Geometry: see drawing. Coordinates: mm, zero at the bounding-box minimum. A direction names the side the tool comes from. Give positions to 0.01 mm unless a question says otherwise; leave off trailing zeros. Write each loop counter-clockwise with the first axis right and the second up, starting at its lowest first coordinate (ties: lowest second). Pieces come first, ordered by that corner, then holes. Notation, with made-up numbers: (81, 74) -> (88, 74) arc R34 cw to (88, 110) -> close; hole circle Ø5 at (-19, -14.75). An arc over 180 degrees is marked (long way). Answer as a JSON object with one key per item and string values. Group by question number.
Item 1: Pull-direction query (Y, two-part tool) for the marked faces 1, 2 and 3; classes: pulls with the +Y half, pulls with the -Y half, needs draft (parallel to the pull), parting line crosses it, or undercut.
Item 2: Section query B-B on y = 14.5. Return the cut outline in (x, z), plus the area to 3 significant figures.
Item 3: Section query D-D on z = 1.75. Return the cut outline in (x, y).
Item 4: First-contact query: pin 1 Ø3 at (y, z) = (7.5, 6.5) entering from +X; pin 2 Ø2.5 at (y, z) = (7, 6.5) entering from -X. Flat tips, straight axial feed; report the tip coordinate or a pass-through.
Item 5: Section query C-C on x = 1.5. Return the cut outline in (y, z).
Item 6: Ray query, probe 1 along Z at (x, y) = (0.65, 7); probe 2 along Z at (x, y) = (3.1, 7); probe 3 along Y at (x, z) = (2.5, 3.5). Return the intervals inside material, ascending. Write a range as from..to.
Item 7: Section query A-A on z = 6.5. Return the cut outline in (x, y).
Item 8: Access query for the marked faces 4 and 5. Directions: +Z, -Z, +X, -X, +Y, -Y. A direction counts if a zero-diameter tool reaches every point of the face in a straight line with its end or side. Return the directions, or none.
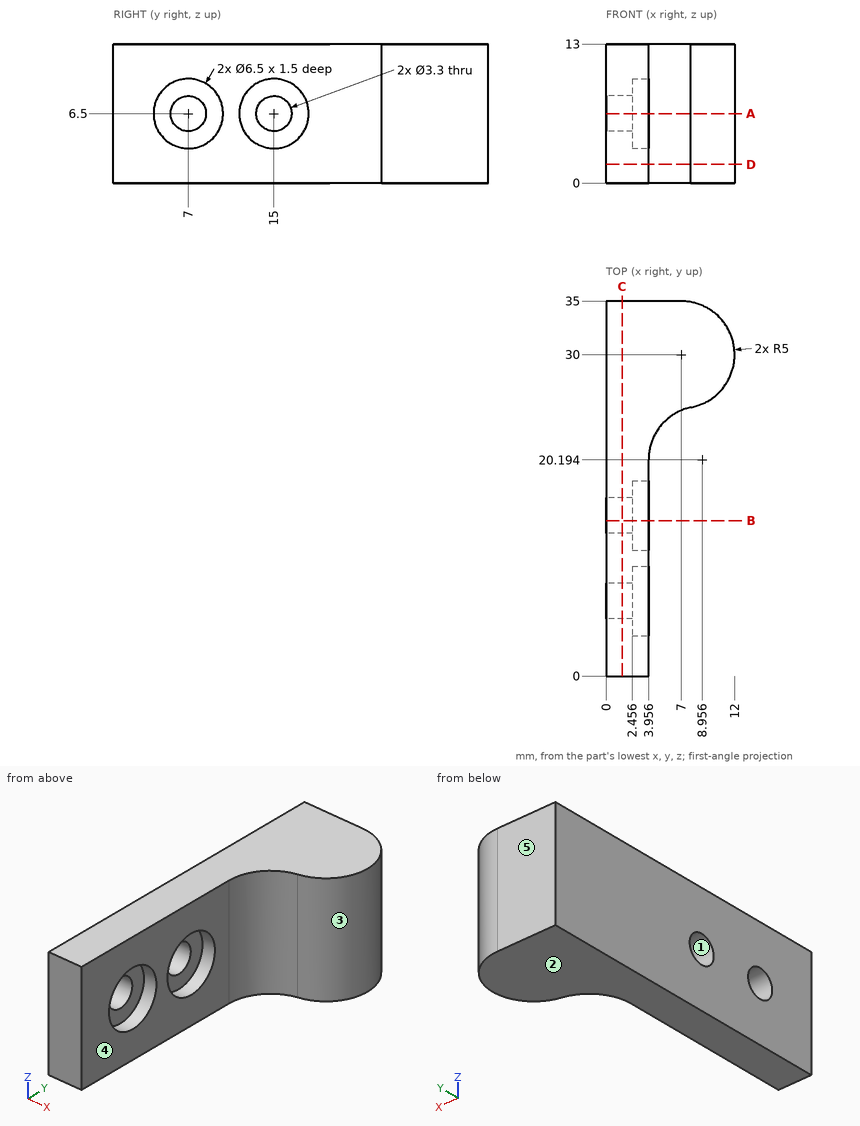
Worked answers:
{
 "1": {"face 1": "undercut", "face 2": "needs draft", "face 3": "parting line crosses it"},
 "2": {"outline": "(0, 0) -> (3.96, 0) -> (3.96, 3.29) -> (2.46, 3.29) -> (2.46, 4.93) -> (0, 4.93) -> close; (0, 8.07) -> (2.46, 8.07) -> (2.46, 9.71) -> (3.96, 9.71) -> (3.96, 13) -> (0, 13) -> close", "area": "34.1 mm^2"},
 "3": {"outline": "(0, 0) -> (3.96, 0) -> (3.96, 20.19) arc R5 cw to (7.91, 25.08) arc R5 ccw to (7, 35) -> (0, 35) -> close"},
 "4": {"pin 1": "x = 2.46", "pin 2": "through"},
 "5": {"outline": "(0, 0) -> (35, 0) -> (35, 13) -> (0, 13) -> close; hole circle Ø3.3 at (7, 6.5); hole circle Ø3.3 at (15, 6.5)"},
 "6": {"probe 1": "0..4.85, 8.15..13", "probe 2": "0..3.25, 9.75..13", "probe 3": "0..5.75, 8.25..13.75, 16.25..35"},
 "7": {"outline": "(0, 0) -> (3.96, 0) -> (3.96, 3.75) -> (2.46, 3.75) -> (2.46, 5.35) -> (0, 5.35) -> close; (0, 8.65) -> (2.46, 8.65) -> (2.46, 10.25) -> (3.96, 10.25) -> (3.96, 11.75) -> (2.46, 11.75) -> (2.46, 13.35) -> (0, 13.35) -> close; (0, 16.65) -> (2.46, 16.65) -> (2.46, 18.25) -> (3.96, 18.25) -> (3.96, 20.19) arc R5 cw to (7.91, 25.08) arc R5 ccw to (7, 35) -> (0, 35) -> close"},
 "8": {"face 4": "+Z, -Z, +X, -Y", "face 5": "+Z, -Z, +X, -X, +Y"}
}
